The listing builds one solid part. Answer for the finished solid, in the listing's coordinates (mm). A direction names the side the tool comes from. Coordinates: 2 decimals unless noted, no trailing zeros. Order: outer loops, then holes, each group sorted by start corner. A loop starts at its lowest first (then second) coordinate and runs counter-clockwise, first axis right, second up. Notation, with made-up numbers: (61, 86) -> (96, 86) arc R22 ccw to (96, 106) -> close; hole circle Ø9 at (-23.75, 63). An arc over 180 degrees is marked (long way). Write item = value, one per line.
from build123d import *

# Parameters (mm, degrees)
SKETCH1_W                      = 629.90984
SKETCH1_H                      = 78.62062
SKETCH1_W_2                    = 32.08
SKETCH1_H_2                    = 32.08
SKETCH1_W_3                    = 32.277504859
SKETCH1_H_3                    = 32.079999999
SKETCH1_W_4                    = 32.400630989
BASE_FLANGE1_DEPTH             = 2.286
EDGE_FLANGE1_STRIP_W           = 13.716
EDGE_FLANGE1_STRIP_H           = 2.286
EDGE_FLANGE1_STRIP_CUT_DEPTH   = 78.62062
EDGE_FLANGE1_STRIP_2_W         = 13.716
EDGE_FLANGE1_STRIP_2_H         = 2.286
EDGE_FLANGE1_STRIP_CUT_2_DEPTH = 78.62062
EDGE_FLANGE1_DEPTH             = 78.62062
EDGE_FLANGE1_BEND_DEPTH        = 78.62062
EDGE_FLANGE2_DEPTH             = 483.60584
CUT_EXTRUDE2_DEPTH             = 719.802540597
CUT_EXTRUDE3_DEPTH             = 891.094678327


# Sheet-metal steps are written as plain solids
with BuildPart() as part:
    # Sketch1 → Base-Flange1 (new body)
    with BuildSketch(Plane.XY):
        with Locations((-571.296524868, -306.535976872)):
            Rectangle(SKETCH1_W, SKETCH1_H)
        with Locations((-839.718644868, -310.649506872)):
            Rectangle(SKETCH1_W_2, SKETCH1_H_2, mode=Mode.SUBTRACT)
        with Locations((-622.144784868, -310.649506872)):
            Rectangle(SKETCH1_W_2, SKETCH1_H_2, mode=Mode.SUBTRACT)
        with Locations((-523.077472438, -310.649506873)):
            Rectangle(SKETCH1_W_3, SKETCH1_H_3, mode=Mode.SUBTRACT)
        with Locations((-305.442049373, -310.649506872)):
            Rectangle(SKETCH1_W_4, SKETCH1_H_2, mode=Mode.SUBTRACT)
    extrude(amount=-BASE_FLANGE1_DEPTH)

    # Edge-Flange1 strip (across the edge) → Edge-Flange1 strip cut (cut)
    with BuildSketch(Plane(origin=(-256.341604868, -345.846286872, 0), x_dir=(-1, 0, 0), z_dir=(0, 1, 0))):
        with Locations((-2.286, -1.143)):
            Rectangle(EDGE_FLANGE1_STRIP_W, EDGE_FLANGE1_STRIP_H)
    extrude(amount=EDGE_FLANGE1_STRIP_CUT_DEPTH, mode=Mode.SUBTRACT)

    # Edge-Flange1 strip 2 (across the edge) → Edge-Flange1 strip cut 2 (cut)
    with BuildSketch(Plane(origin=(-886.251444868, -267.225666872, 0), x_dir=(1, 0, 0), z_dir=(0, -1, 0))):
        with Locations((-2.286, -1.143)):
            Rectangle(EDGE_FLANGE1_STRIP_2_W, EDGE_FLANGE1_STRIP_2_H)
    extrude(amount=EDGE_FLANGE1_STRIP_CUT_2_DEPTH, mode=Mode.SUBTRACT)

    # Edge-Flange1 section (across the edge) → Edge-Flange1 (add)
    with BuildSketch(Plane(origin=(-256.341604868, -345.846286872, 0), x_dir=(-1, 0, 0), z_dir=(0, 1, 0))):
        with BuildLine():
            Line((0, 2.286), (0, 16.764))
            Line((0, 16.764), (2.286, 16.764))
            Line((2.286, 16.764), (2.286, 2.286))
            ThreePointArc((2.286, 2.286), (2.955553898, 0.669553898), (4.572, 0))
            Line((4.572, 0), (4.572, -2.286))
            ThreePointArc((4.572, -2.286), (1.339107796, -0.946892204), (0, 2.286))
        make_face()
    extrude(amount=EDGE_FLANGE1_DEPTH)

    # Edge-Flange1 section 2 (across the edge) → Edge-Flange1 bend (add)
    with BuildSketch(Plane(origin=(-886.251444868, -267.225666872, 0), x_dir=(1, 0, 0), z_dir=(0, -1, 0))):
        with BuildLine():
            Line((0, 2.286), (0, 16.764))
            Line((0, 16.764), (2.286, 16.764))
            Line((2.286, 16.764), (2.286, 2.286))
            ThreePointArc((2.286, 2.286), (2.955553898, 0.669553898), (4.572, 0))
            Line((4.572, 0), (4.572, -2.286))
            ThreePointArc((4.572, -2.286), (1.339107796, -0.946892204), (0, 2.286))
        make_face()
    extrude(amount=EDGE_FLANGE1_BEND_DEPTH)

    # Edge-Flange2 section (across the edge) → Edge-Flange2 (add)
    with BuildSketch(Plane(origin=(-329.493604868, -264.939666872, 0), x_dir=(0, -1, 0), z_dir=(-1, 0, 0))):
        with BuildLine():
            Line((-2.286, 2.286), (-2.286, 16.764))
            Line((-2.286, 16.764), (0, 16.764))
            Line((0, 16.764), (0, 2.286))
            ThreePointArc((0, 2.286), (0.669553898, 0.669553898), (2.286, 0))
            Line((2.286, 0), (2.286, -2.286))
            ThreePointArc((2.286, -2.286), (-0.946892204, -0.946892204), (-2.286, 2.286))
        make_face()
    extrude(amount=EDGE_FLANGE2_DEPTH)

    # Sketch26 → Cut-Extrude2 (cut, through all)
    with BuildSketch(Plane.ZY.offset(886.251444868)):
        with BuildLine():
            Line((12.575, -285.610821872), (12.575, -288.150821872))
            ThreePointArc((12.575, -288.150821872), (9.525, -291.200821872), (6.475, -288.150821872))
            Line((6.475, -288.150821872), (6.475, -285.610821872))
            ThreePointArc((6.475, -285.610821872), (9.525, -282.560821872), (12.575, -285.610821872))
        make_face()
        with BuildLine():
            Line((12.575, -327.461131872), (12.575, -324.921131872))
            ThreePointArc((12.575, -324.921131872), (9.525, -321.871131872), (6.475, -324.921131872))
            Line((6.475, -324.921131872), (6.475, -327.461131872))
            ThreePointArc((6.475, -327.461131872), (9.525, -330.511131872), (12.575, -327.461131872))
        make_face()
    extrude(amount=-CUT_EXTRUDE2_DEPTH, mode=Mode.SUBTRACT)

    # Sketch27 → Cut-Extrude3 (cut, through all)
    with BuildSketch(Plane.XZ.offset(264.939666872)):
        with BuildLine():
            Line((-753.918714868, 12.575), (-751.378714868, 12.575))
            ThreePointArc((-751.378714868, 12.575), (-748.328714868, 9.525), (-751.378714868, 6.475))
            Line((-751.378714868, 6.475), (-753.918714868, 6.475))
            ThreePointArc((-753.918714868, 6.475), (-756.968714868, 9.525), (-753.918714868, 12.575))
        make_face()
        with BuildLine():
            Line((-630.477254868, 12.575), (-633.017254868, 12.575))
            ThreePointArc((-633.017254868, 12.575), (-636.067254868, 9.525), (-633.017254868, 6.475))
            Line((-633.017254868, 6.475), (-630.477254868, 6.475))
            ThreePointArc((-630.477254868, 6.475), (-627.427254868, 9.525), (-630.477254868, 12.575))
        make_face()
        with BuildLine():
            Line((-388.674334868, 12.575), (-391.214334868, 12.575))
            ThreePointArc((-391.214334868, 12.575), (-394.264334868, 9.525), (-391.214334868, 6.475))
            Line((-391.214334868, 6.475), (-388.674334868, 6.475))
            ThreePointArc((-388.674334868, 6.475), (-385.624334868, 9.525), (-388.674334868, 12.575))
        make_face()
        with BuildLine():
            Line((-512.115794868, 12.575), (-509.575794868, 12.575))
            ThreePointArc((-509.575794868, 12.575), (-506.525794868, 9.525), (-509.575794868, 6.475))
            Line((-509.575794868, 6.475), (-512.115794868, 6.475))
            ThreePointArc((-512.115794868, 6.475), (-515.165794868, 9.525), (-512.115794868, 12.575))
        make_face()
    extrude(amount=-CUT_EXTRUDE3_DEPTH, mode=Mode.SUBTRACT)


solid = part.part
Q1. The mould has two halves that part along X. Classify faces 1 (the face through (-256.342, -307, 9)), 2 (the face through (-576, -306, 0)), 3 (the face through (-285, -267.226, -1)): released by +X, released by -X, zero draft, split by the parting line, or undercut.
The answers:
face_1 = released by +X
face_2 = undercut
face_3 = zero draft
Q2. A tool of negligible diameter and unlimited length cuts with its end or side. For faces 4 (the face through (-857.6, -267.226, -0.5)), 5 (the face through (-568, -262.654, 9)), 6 (the face through (-258.628, -307, 10)), 7 (the face through (-568, -264.94, 10)), from which of +Z, -Z, +X, -X, +Y, -Y can it reach the whole face along a straight path? Write none if from no direction.
The answers:
face_4 = +Z, -Z, -X, +Y
face_5 = +Z, -Z, +X, -X, +Y
face_6 = +Z, +Y, -Y
face_7 = +Z, +X, -X, -Y
Q3. Section A-A, the plane y = -301.5 is taken. Give the vertices of the cut face in (x, z), plus the area to 3 significant figures.
The answers:
outline = (-886.25, 2.29) arc R4.57 ccw to (-881.68, -2.29) -> (-855.76, -2.29) -> (-855.76, 0) -> (-881.68, 0) arc R2.29 cw to (-883.97, 2.29) -> (-883.97, 16.76) -> (-886.25, 16.76) -> close; (-823.68, -2.29) -> (-638.18, -2.29) -> (-638.18, 0) -> (-823.68, 0) -> close; (-606.1, -2.29) -> (-539.22, -2.29) -> (-539.22, 0) -> (-606.1, 0) -> close; (-506.94, -2.29) -> (-321.64, -2.29) -> (-321.64, 0) -> (-506.94, 0) -> close; (-289.24, -2.29) -> (-260.91, -2.29) arc R4.57 ccw to (-256.34, 2.29) -> (-256.34, 16.76) -> (-258.63, 16.76) -> (-258.63, 2.29) arc R2.29 cw to (-260.91, 0) -> (-289.24, 0) -> close
area = 1,220 mm2
Q4. Each of these flat-tipped pins is pushed along its axis until it touches: pin 1 Ø8 at (x, y) = (-613, -319) entering from -Z; pin 2 Ø1.1 at (y, z) = (-308, -1) entering from -X; pin 3 Ø1.1 at (y, z) = (-309, -1.5) entering from -X; pin 4 Ø10 at (x, z) = (-720.5, 1.5) entering from +Y. Where does it stop, or does it pass through?
The answers:
pin_1 = through
pin_2 = -885.34
pin_3 = -884.91
pin_4 = -262.65
Q5. Section B-B, the plane x = -733.5 is taken. Give the vertices of the cut face in (y, z), plus the area to 3 significant figures.
The answers:
outline = (-345.85, -2.29) -> (-267.23, -2.29) arc R4.57 ccw to (-262.65, 2.29) -> (-262.65, 16.76) -> (-264.94, 16.76) -> (-264.94, 2.29) arc R2.29 cw to (-267.23, 0) -> (-345.85, 0) -> close
area = 225 mm2
Q6. Find the intervals of material crossed by line 1 along X through (y, z) = (-302, 6.5); line 2 along X through (y, z) = (-338.5, 2); line 3 along Z through (x, y) = (-549.5, -291), in increasing order.
The answers:
line_1 = -886.25 to -883.97, -258.63 to -256.34
line_2 = -886.24 to -883.95, -258.65 to -256.35
line_3 = -2.29 to 0
